Check sheet for the modelled part. Datum: model origin and axes. Units: mm. A direction names the side the tool comes from. Coordinates: 2 decimals unless noted, no trailing zeros. Loops run counter-clockwise (first coordinate to the right, second up) from the corner with the lowest first, then second, coordinate; pieces in that order, holes last. Notation, with made-up numbers: (39.25, 3.25) - (60.25, 3.25) arc R10 ccw to (60.25, 21.25) - close; hole circle Ø1 at (21, -4.75). An arc over 180 degrees is marked (long way). Use a Markdown table: item, result. Add a question column.
1) Sectioned sample at A-A, the plane y = -7.25. Enter the section's corners in (x, z).
2) Sectioned sample at D-D, the plane y = -12. Enter the section's corners in (x, z), then the cut area to 3 significant figures.
3) Sectioned sample at C-C, the plane z = 0.55. Enter the section's corners in (x, y), then the cut area to 3 significant figures.
4) Sectioned sample at B-B, the plane x = 7. Enter the section's corners in (y, z), then the cut area to 3 significant figures.
5) Draft check along X on faces 3 (the flat face through (7, 2.159, 2)), 4 (the flat face through (4.722, -7, 2)), 5 (the cylindrical face through (7.66, 1.06, 2.69)). Enter one of: pulls with the +X half, pulls with the -X half, needs draft (parallel to the pull), parting line crosses it, or undercut.
6) Thickness scan on line 1 (X direction, y = -8.25, z = 2.35); line 2 (Y direction, x = 12.5, z = 0.4); line 3 (Y direction, x = 7, z = 0.65). Record the ranges inside material, lowest first.
7) Tool access check on faces 1 (the flat face through (9.122, -7, 2)), 2 (the flat face through (13.843, -7, 2)). Record the directions out of +Z, -Z, +X, -X, +Y, -Y that give a thin tool (end or side, any length) a straight path to the whole face; none if there is none.
from build123d import *

# Parameters (mm, degrees)
SKETCH1_W           = 13.843
SKETCH1_H           = 13.843
BOSS_EXTRUDE1_DEPTH = 4.7625
SKETCH2_R           = 0.8001
BOSS_EXTRUDE2_DEPTH = 2.159
CUT_EXTRUDE1_DEPTH  = 8.001


with BuildPart() as part:
    # Sketch1 → Boss-Extrude1 (new body)
    with BuildSketch(Plane.XY):
        with Locations((6.9215, -6.9215)):
            Rectangle(SKETCH1_W, SKETCH1_H)
    extrude(amount=BOSS_EXTRUDE1_DEPTH)

    # Sketch2 → Boss-Extrude2 (add)
    with BuildSketch(Plane(origin=(0, 0, 0), x_dir=(1, 0, 0), z_dir=(0, 1, 0))):
        with Locations((6.9215, -2.38125)):
            Circle(SKETCH2_R)
    extrude(amount=BOSS_EXTRUDE2_DEPTH)

    # Sketch3 → Cut-Extrude1 (cut)
    with BuildSketch(Plane(origin=(0, 0, 0), x_dir=(-1, 0, 0), z_dir=(0, 0, -1))):
        with BuildLine():
            Line((-9.1215, -10.0965), (-9.1215, -3.7465))
            ThreePointArc((-9.1215, -3.7465), (-6.9215, -1.5465), (-4.7215, -3.7465))
            Line((-4.7215, -3.7465), (-4.7215, -10.0965))
            ThreePointArc((-4.7215, -10.0965), (-6.9215, -12.2965), (-9.1215, -10.0965))
        make_face()
    extrude(amount=-CUT_EXTRUDE1_DEPTH, mode=Mode.SUBTRACT)


solid = part.part
Solved:
| question | item | result |
|---|---|---|
| 1 | outline | (0, 0) - (4.72, 0) - (4.72, 4.76) - (0, 4.76) - close; (9.12, 0) - (13.84, 0) - (13.84, 4.76) - (9.12, 4.76) - close |
| 2 | outline | (0, 0) - (5.82, 0) - (5.82, 4.76) - (0, 4.76) - close; (8.02, 0) - (13.84, 0) - (13.84, 4.76) - (8.02, 4.76) - close |
| 2 | area | 55.4 mm2 |
| 3 | outline | (0, -13.84) - (13.84, -13.84) - (13.84, 0) - (0, 0) - close; hole (4.72, -10.1) arc R2.2 ccw to (9.12, -10.1) - (9.12, -3.75) arc R2.2 ccw to (4.72, -3.75) - close |
| 3 | area | 148 mm2 |
| 4 | outline | (-13.84, 0) - (-12.3, 0) - (-12.3, 4.76) - (-13.84, 4.76) - close; (-1.55, 0) - (0, 0) - (0, 1.59) - (2.16, 1.59) - (2.16, 3.18) - (0, 3.18) - (0, 4.76) - (-1.55, 4.76) - close |
| 4 | area | 18.2 mm2 |
| 5 | face 3 | needs draft |
| 5 | face 4 | undercut |
| 5 | face 5 | parting line crosses it |
| 6 | line 1 | x = 0 to 4.72, 9.12 to 13.84 |
| 6 | line 2 | y = -13.84 to 0 |
| 6 | line 3 | y = -13.84 to -12.3, -1.55 to 0 |
| 7 | face 1 | +Z, -Z |
| 7 | face 2 | +Z, -Z, +X, +Y, -Y |
